Geometry: final body of the model. Coordinates: model frame, mm. A direction names the side the tool comes from. Give positions to 0.01 mm unless a question says otherwise; leave off trailing zeros. Write each loop counter-clockwise with the first axis right and the second up, starting at its lowest first coordinate (ties: lowest second). Pieces come first, ordered by that corner, then holes.
```python
from build123d import *

# Parameters (mm, degrees)
CROQUIS1_W                       = 594
CROQUIS1_H                       = 19.095477387
BRIDA_BASE1_DEPTH                = 6.35
PLIEGUE_CROQUIZADO1_DEPTH        = 19.095477387
PLIEGUE_CROQUIZADO1_2_DEPTH      = 19.095477387
TALADRO_DE_MARGEN_PARA_M51_D     = 5.5
TALADRO_DE_MARGEN_PARA_M52_D     = 5.5
TALADRO_DE_MARGEN_PARA_M52_DEPTH = 6.35


with BuildPart() as part:
    # Brida base1: sheet metal written as solids
    # Croquis1 → Brida base1 (new body)
    with BuildSketch(Plane.XY):
        with Locations((58.84427983, 9.547738694)):
            Rectangle(CROQUIS1_W, CROQUIS1_H)
    extrude(amount=-BRIDA_BASE1_DEPTH)

    # Pliegue croquizado1: read off the stored shape, not the designer's step
    # Pliegue croquizado1 outline → Pliegue croquizado1 (cut)
    with BuildSketch(Plane(origin=(0, 0, 0), x_dir=(1, 0, 0), z_dir=(0, 1, 0))):
        with BuildLine():
            ThreePointArc((-142.131770672, 0), (-139.826968461, 4.528373368), (-135.083556714, 6.35))
            Line((-135.083556714, 6.35), (-238.15572017, 6.35))
            Line((-238.15572017, 6.35), (-238.15572017, 0))
            Line((-238.15572017, 0), (-142.131770672, 0))
        make_face()
        with BuildLine():
            Line((355.84427983, 6.35), (137.772116374, 6.35))
            ThreePointArc((137.772116374, 6.35), (142.515528121, 4.528373367), (144.820330332, 0))
            Line((144.820330332, 0), (355.84427983, 0))
            Line((355.84427983, 0), (355.84427983, 6.35))
        make_face()
    extrude(amount=PLIEGUE_CROQUIZADO1_DEPTH, mode=Mode.SUBTRACT)

    # Pliegue croquizado1 2 outline → Pliegue croquizado1 2 (add)
    with BuildSketch(Plane(origin=(0, 0, 0), x_dir=(1, 0, 0), z_dir=(0, 1, 0))):
        with BuildLine():
            Line((-135.083556714, 0), (-142.131770672, 0))
            ThreePointArc((-142.131770672, 0), (-142.160553697, -0.367800241), (-142.170156714, -0.7366))
            Line((-142.170156714, -0.7366), (-142.170156714, -97.664436544))
            Line((-142.170156714, -97.664436544), (-135.820156714, -97.664436544))
            Line((-135.820156714, -97.664436544), (-135.820156714, -0.7366))
            ThreePointArc((-135.820156714, -0.7366), (-135.604411569, -0.215745145), (-135.083556714, 0))
        make_face()
        with BuildLine():
            ThreePointArc((144.858716374, -0.7366), (144.849113357, -0.367800241), (144.820330332, 0))
            Line((144.820330332, 0), (137.772116374, 0))
            ThreePointArc((137.772116374, 0), (138.292971229, -0.215745145), (138.508716374, -0.7366))
            Line((138.508716374, -0.7366), (138.508716374, -212.664436544))
            Line((138.508716374, -212.664436544), (144.858716374, -212.664436544))
            Line((144.858716374, -212.664436544), (144.858716374, -0.7366))
        make_face()
    extrude(amount=PLIEGUE_CROQUIZADO1_2_DEPTH)

    # Taladro de margen para M51 (through all)
    with Locations(Plane(origin=(144.858716374, 0, 0), x_dir=(0, 0, -1), z_dir=(1, 0, 0))):
        with Locations((-192.664436544, 9.547738693), (-132.664436544, 9.547738693)):
            Hole(TALADRO_DE_MARGEN_PARA_M51_D / 2)

    # Taladro de margen para M52
    with Locations(Plane(origin=(-135.820156714, 0, 0), x_dir=(0, 0, -1), z_dir=(1, 0, 0))):
        with Locations((-87.664436544, 8.935987286), (-27.664436544, 8.935987286)):
            Hole(TALADRO_DE_MARGEN_PARA_M52_D / 2, depth=TALADRO_DE_MARGEN_PARA_M52_DEPTH)


solid = part.part
```
Item 1: Reachability of faces 5 (the face through (141.639, 9.669, 129.917)), 6 (the face through (-1, 10, -6.35)), 7 (the face through (-139.04, 9.057, 84.917)), 8 (the face through (-139, 9, 97.664)), 9 (the face through (-135.82, 9, 50)) from +Z, -Z, +X, -X, +Y, -Y: full face, straight path, thin tool, end or side. Return the list, or none.
Found:
face 5: +X, -X
face 6: -Z, +X, -X, +Y, -Y
face 7: -X
face 8: +Z, -X, +Y, -Y
face 9: +Z, +Y, -Y
Item 2: Pin query (flat end, axial travel): pin 1 Ø5.5 at (x, y) = (-64, 12) entering from +Z; pin 2 Ø7 at (y, z) = (9.55, 192.66) entering from +X; pin 3 Ø7 at (x, y) = (-138.5, 6) entering from +Z; pin 4 Ø3.5 at (y, z) = (9.55, 132.66) entering from +X. Return the tip coordinate at first contact, or that it passes through.
Found:
pin 1: stops at z = 0
pin 2: stops at x = 144.86
pin 3: stops at z = 97.66
pin 4: passes through
Item 3: Section C-C, the plane x = 53. Return the cut outline in (y, z), plus the area to 3 significant figures.
Found:
outline: (0, -6.35) - (19.1, -6.35) - (19.1, 0) - (0, 0) - close
area: 121 mm2
Item 4: Line query: L1, parallel to X at y = 9.5, z = 62; L2, parallel to X at y = 10, z = 115; L3, parallel to Z at x = 39, y = 13.75. Output: solid intervals per line, ascending.
Found:
L1: x = -142.17 to -135.82, 138.51 to 144.86
L2: x = 138.51 to 144.86
L3: z = -6.35 to 0
Item 5: Pull-direction query (X, two-part tool) for faces 1 (the face through (144.859, 9, 108)), 2 (the face through (138.509, 9, 105)), 3 (the face through (-139.04, 9.76, 30.29)), 4 (the face through (-142.17, 9, 49)); classes: +X half, -X half, draft (parallel to the pull), parting line (faces both ways), or undercut.
Found:
face 1: +X half
face 2: undercut
face 3: draft
face 4: -X half
Item 6: Section B-B, the plane z = 178. Return the cut outline in (x, y).
Found:
outline: (138.51, 0) - (144.86, 0) - (144.86, 19.1) - (138.51, 19.1) - close
Item 7: Section A-A, the plane z = 15.5. Return the cut outline in (x, y), plus the area to 3 significant figures.
Found:
outline: (-142.17, 0) - (-135.82, 0) - (-135.82, 19.1) - (-142.17, 19.1) - close; (138.51, 0) - (144.86, 0) - (144.86, 19.1) - (138.51, 19.1) - close
area: 243 mm2
